Design review of the part built by this model. Coordinates are the model's own, in mm. Round coordinates to 2 decimals unless told otherwise and drop trailing zeros. Order: outer loops, then holes, each group sorted by start corner. A loop starts at its lowest first (then second) coordinate and runs counter-clockwise, first axis right, second up. Notation, with made-up numbers: (53.5, 68) - (96.5, 68) arc R25 cw to (96.5, 90) - close; hole circle Ø8 at (82, 17). An arc over 180 degrees is marked (long way). Write item = value, one per line.
Autodesk Inventor part; units mm, degrees
ref_plane "YZ Plane" through (0, 0, 0) normal (1, 0, 0) x (0, 1, 0)
ref_plane "XZ Plane" through (0, 0, 0) normal (0, 1, 0) x (-1, 0, 0)
ref_plane "XY Plane" through (0, 0, 0) normal (0, 0, 1) x (1, 0, 0)
sketch "Sketch1" plane through (0, 0, 0) normal (1, 0, 0) x (0, 1, 0)
  circle A0 centre (0, 0) radius 26
  circle A1 centre (0, 0) radius 17.5
  line L0 (9.2645, 0) -> (-12.3906, 0) construction
  circle A2 centre (0, 0) radius 21.5 construction
  line L1 (0, 0) -> (0, -36.6713) construction
  point P0 (0, -21.5)
  point P1 (18.6195, 10.75)
  point P2 (-18.6195, 10.75)
  dimension "d1" = 43
  dimension "d0" = 35
  dimension "d2" = 52
  dimension "d5" = 360
extrude "Extrusion1" add sketch "Sketch1" along normal blind 6
hole "Hole1" at (0, 0, -21.5) at (0, 18.6195, 10.75) at (0, -18.6195, 10.75) direction (1, 0, 0) diameter 3 depth 10 tip angle 118
properties part number "Soporte2_Rodamientos"
Item 1: Insertion check: P1, Ø1, axis at x = 3, z = -6, coming from the +Y side; P2, Ø2, axis at x = 3.5, z = 5.5, coming from the -Y side; P3, Ø2, axis at x = 1, y = -4.5, coming from the +Z side. Each pin has a flat end and moves straight along its axis. Give the tip position at first contact, or say it passes through.
Data:
P1 = 25.41
P2 = -25.61
P3 = 25.76
Item 2: For line 1 along Z through (x, y) = (1.7, 0); line 2 along Y through (x, z) = (2.45, 9.5); line 3 along Y through (x, z) = (2.45, 10.75), list the stretches that pass through material, from the lowest coordinate up. Write a range as [from, to].
Data:
line_1 = [-26, -23], [-20, -17.5], [17.5, 26]
line_2 = [-24.2, -19.45], [-17.79, -14.7], [14.7, 17.79], [19.45, 24.2]
line_3 = [-23.67, -20.12], [-17.12, -13.81], [13.81, 17.12], [20.12, 23.67]
Item 3: Take a section at C-C, the plane z = 10.75. State the section outline as (x, y) points, and give its area (3 significant figures).
Data:
outline = (0, -23.67) - (6, -23.67) - (6, -20.12) - (0, -20.12) - close; (0, -17.12) - (6, -17.12) - (6, -13.81) - (0, -13.81) - close; (0, 13.81) - (6, 13.81) - (6, 17.12) - (0, 17.12) - close; (0, 20.12) - (6, 20.12) - (6, 23.67) - (0, 23.67) - close
area = 82.4 mm2
Item 4: The part is to be moulded in two halves that separate along Y. For faces 1 (the face through (2.958, -20.633, 15.821)), 2 (the face through (6, 17, -5)), 3 (the face through (3.042, 20.084, 10.425)), say which applies: +Y half, -Y half, draft (parallel to the pull), parting line (faces both ways), or undercut.
Data:
face_1 = parting line
face_2 = draft
face_3 = undercut
Item 5: Take a section at D-D, the plane y = 15. State the section outline as (x, z) points.
Data:
outline = (0, -21.24) - (6, -21.24) - (6, -9.01) - (0, -9.01) - close; (0, 9.01) - (6, 9.01) - (6, 21.24) - (0, 21.24) - close
Item 6: Take a section at A-A, the plane y = 0. State the section outline as (x, z) points, and give its area (3 significant figures).
Data:
outline = (0, -26) - (6, -26) - (6, -23) - (0, -23) - close; (0, -20) - (6, -20) - (6, -17.5) - (0, -17.5) - close; (0, 17.5) - (6, 17.5) - (6, 26) - (0, 26) - close
area = 84.0 mm2
Item 7: Take a section at B-B, the plane z = 0. State the section outline as (x, y) points, and give its area (3 significant figures).
Data:
outline = (0, -26) - (6, -26) - (6, -17.5) - (0, -17.5) - close; (0, 17.5) - (6, 17.5) - (6, 26) - (0, 26) - close
area = 102 mm2
